Here's the drawing with two shaded views (mm, measured from the low corner). I have some questions. A direction names the side the tool comes from. Coordinates: 2 decimals unless noted, no trailing zeros. Loops run counter-clockwise (first coordinate to the right, second up) from the corner with the lowest first, then second, coordinate; pieces in that order, holes last.
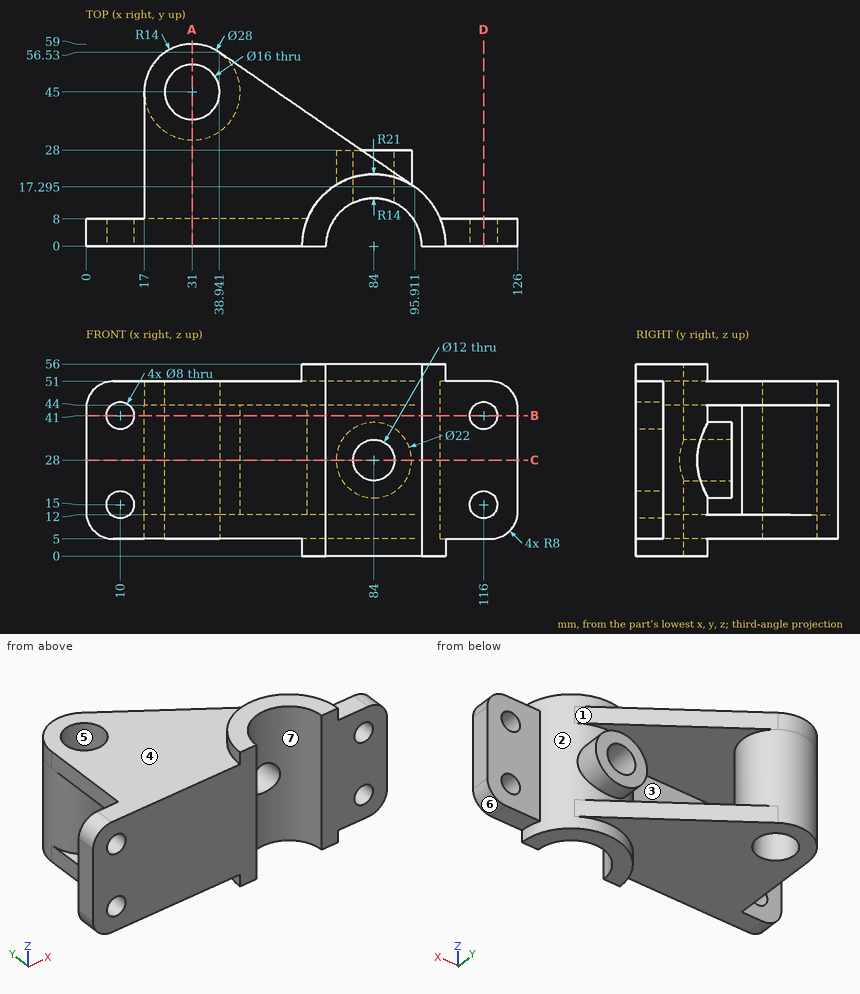
(1) If I drill on probe 1 along Y at (x, z) = (31, 39); probe 2 along Z at (x, y) = (44, 39); probe 3 along X at (y, z) = (5, 41), over which ranges is the centre line in solid material (lowest first)?
Check values:
probe 1: y = 0 to 8, 31 to 37, 53 to 59
probe 2: z = 5 to 12, 44 to 51
probe 3: x = 0 to 6, 14 to 70.92, 97.08 to 112, 120 to 126
(2) If we mould it in two halves opening along X, with no side actions, what happens to the marked faces 4, 5, 6 and 7? For each: released by +X, released by -X, zero draft, split by the parting line, or undercut.
Check values:
face 4: zero draft
face 5: undercut
face 6: released by +X
face 7: undercut
(3) I'm going to push flat-ended pins straight in: pin 1 (14.5 mm diameter, centred on x = 42, y = 24.5, fed in from +Z); pin 2 (3 mm diameter, centred on x = 40.5, z = 49.5, fed in from +Y); pin 3 (6 mm diameter, centred on y = 18.5, z = 35, fed in from -X); pin 4 (7 mm diameter, centred on x = 10, z = 15, fed in from +Y) (3 decimals). Where does each tip first touch, or does it pass through?
Check values:
pin 1: stops at z = 51
pin 2: stops at y = 56.49
pin 3: stops at x = 69.83
pin 4: passes through
(4) I want a section at C-C on z = 28. Write out the boundary of the cut face in (x, y), then the cut area to 3 significant figures.
Check values:
outline: (0, 0) - (70, 0) arc R14 cw to (78, 12.65) - (78, 28) - (73, 28) - (73, 17.89) arc R21 ccw to (64.58, 8) - (0, 8) - close; circle Ø28 at (31, 45); (90, 12.65) arc R14 cw to (98, 0) - (126, 0) - (126, 8) - (103.42, 8) arc R21 ccw to (95, 17.89) - (95, 28) - (90, 28) - close; hole circle Ø16 at (31, 45)
area: 1,480 mm2
(5) I want a section at A-A on x = 31. Write out the boundary of the cut face in (y, z).
Check values:
outline: (0, 5) - (37, 5) - (37, 51) - (0, 51) - close; (53, 5) - (59, 5) - (59, 51) - (53, 51) - close; hole (8, 12) - (31, 12) - (31, 44) - (8, 44) - close
(6) I want a section at D-D on x = 116. Write out the boundary of the cut face in (y, z), then the cut area to 3 significant figures.
Check values:
outline: (0, 5) - (8, 5) - (8, 11) - (0, 11) - close; (0, 19) - (8, 19) - (8, 37) - (0, 37) - close; (0, 45) - (8, 45) - (8, 51) - (0, 51) - close
area: 240 mm2
(7) Which directions (+Z, -Z, +X, -X, +Y, -Y) give clear straight access to the entire face, cutting with the end or side of a thin tool? Please do the marked faces 1, 2 and 3.
Check values:
face 1: +Z, +X, +Y
face 2: +Y
face 3: -X
(8) I want a section at B-B on z = 41. Write out the boundary of the cut face in (x, y).
Check values:
outline: (0, 0) - (6, 0) - (6, 8) - (0, 8) - close; (14, 0) - (70, 0) arc R14 cw to (98, 0) - (112, 0) - (112, 8) - (103.42, 8) arc R21 ccw to (64.58, 8) - (14, 8) - close; circle Ø28 at (31, 45); (120, 0) - (126, 0) - (126, 8) - (120, 8) - close; hole circle Ø16 at (31, 45)
